Autodesk Inventor part; units mm, degrees
ref_plane "YZ Plane" through (0, 0, 0) normal (1, 0, 0) x (0, 1, 0)
ref_plane "XZ Plane" through (0, 0, 0) normal (0, 1, 0) x (-1, 0, 0)
ref_plane "XY Plane" through (0, 0, 0) normal (0, 0, 1) x (1, 0, 0)
sketch "Sketch1" plane through (0, 0, 0) normal (0, 1, 0) x (-1, 0, 0)
  line L0 (0, 0) -> (7, 0)
  line L1 (7, -23.495) -> (0, -23.495)
  line L2 (-11.75, -2) -> (-11.75, -21.5)
  line L3 (-11.75, -9.75) -> (-10, -9.75)
  line L4 (-10, -2) -> (-10, -21.5)
  line L5 (-11.75, -0.1283) -> (-10, -0.1283)
  line L6 (-10, -2) -> (-10, -6)
  line L7 (-11.75, -6) -> (-13.75, -6)
  line L8 (-13.75, -6) -> (-13.75, 0)
  line L9 (-10, -6) -> (-8, -6)
  line L10 (-8, -6) -> (-8, 0)
  line L11 (-8, 0) -> (-13.75, 0)
  line L12 (-10, -21.5) -> (-10, -17.5)
  line L13 (-10, -17.5) -> (-8, -17.5)
  line L14 (-8, -17.5) -> (-8, -23.5)
  line L15 (-10, -2) -> (-11.75, -2)
  line L16 (-11.75, -6) -> (-11.75, -2)
  line L17 (-10, -21.5) -> (-11.75, -21.5)
  line L18 (-11.75, -21.5) -> (-11.75, -17.5)
  line L19 (-11.75, -17.5) -> (-13.75, -17.5)
  line L20 (-13.75, -17.5) -> (-13.75, -23.5)
  line L21 (-13.75, -23.5) -> (-8, -23.5)
  line L22 (-0.01, -3.75) -> (7, -3.75)
  line L23 (-8, -6) -> (-0.01, -3.75)
  line L24 (-8, 0) -> (7, 0)
  line L25 (7, 0) -> (7, -3.75)
  line L26 (-8, -23.5) -> (7, -23.5)
  line L27 (7, -23.5) -> (7, -19.75)
  line L28 (7, -19.75) -> (-0.01, -19.75)
  line L29 (-8, -17.5) -> (-0.01, -19.75)
  line L30 (7, -23.5) -> (0, -23.5)
  line L31 (0, -23.5) -> (0, 0)
  line L32 (0, 0) -> (7, 0)
  line L33 (7, 0) -> (7, -23.5)
  line L34 (-10, -21.5) -> (-9.75, -21.5)
  line L35 (-9.75, -21.5) -> (-9.75, -17.5)
  line L36 (-9.75, -17.5) -> (-10, -17.5)
  line L37 (-10, -17.5) -> (-10, -21.5)
  line L38 (-11.75, -17.5) -> (-12, -17.5)
  line L39 (-12, -17.5) -> (-12, -21.5)
  line L40 (-12, -21.5) -> (-11.75, -21.5)
  line L41 (-11.75, -21.5) -> (-11.75, -17.5)
  line L42 (-10, -6) -> (-9.75, -6)
  line L43 (-9.75, -6) -> (-9.75, -2)
  line L44 (-9.75, -2) -> (-10, -2)
  line L45 (-10, -2) -> (-10, -6)
  line L46 (-11.75, -6) -> (-12, -6)
  line L47 (-12, -6) -> (-12, -2)
  line L48 (-12, -2) -> (-11.75, -2)
  line L49 (-11.75, -2) -> (-11.75, -6)
  dimension "d0" = 23.495
  dimension "d1" = 7
  dimension "d2" = 4
  dimension "d3" = 2
  dimension "d4" = 6
  dimension "d5" = 2
  dimension "d6" = 4
  dimension "d7" = 2
  dimension "d8" = 6
  dimension "d9" = 2
  dimension "d10" = 15
  dimension "d11" = 15
  dimension "d12" = 0.25
  dimension "d13" = 0.25
  dimension "d14" = 0.25
  dimension "d15" = 0.25
extrude "Extrusion1" add sketch "Sketch1" along normal blind 14.5 contours L31 L22 L23 L10 L24 | L0 L25 L22 L31 | L10 L9 L43 L44 L15 L48 L47 L7 L8 L11 | L22 L33 L28 L31 | L31 L26 L14 L29 L28 | L28 L27 L1 L31 | L1 L27 L26 L31 | L14 L21 L20 L19 L39 L40 L17 L34 L35 L13
sketch "Sketch2" plane through (-7, 0, -23.5) normal (-1, 0, 0) x (0, 0, 1)
  line L0 (23.5, 0) -> (19.75, 0)
  line L1 (19.75, 0) -> (3.75, 0)
  line L2 (19.75, 0) -> (19.75, 14.5)
  line L3 (19.75, 0) -> (19.75, 14.5)
  line L4 (6, 0) -> (0, 0)
  line L5 (0, 0) -> (3.75, 0)
  line L6 (3.75, 0) -> (3.75, 14.5)
  line L7 (3.75, 0) -> (3.75, 14.5)
  line L8 (3.75, 0) -> (19.75, 0)
  line L9 (19.75, 0) -> (19.75, 14.5)
  line L10 (19.75, 14.5) -> (3.75, 14.5)
  line L11 (3.75, 14.5) -> (3.75, 0)
  dimension "d18" = 3.75
  dimension "d19" = 3.75
extrude "Extrusion2" add sketch "Sketch2" along normal blind 30
sketch "Sketch3" plane through (0, 0, 0) normal (0, -1, 0) x (1, 0, 0)
  line L0 (-37, -19.75) -> (-37, -3.75)
  circle A0 centre (-37, -11.75) radius 10.75
  point P0 (0, 0)
  dimension "d22" = 21.5
extrude "Extrusion3" add sketch "Sketch3" against normal blind 14.5
sketch "Sketch4" plane through (0, 0, 0) normal (0, -1, 0) x (1, 0, 0)
  arc A0 (-29.8193, -3.75) -> (-29.8193, -19.75) centre (-37, -11.75) ccw
  circle A1 centre (-37, -11.75) radius 10
  point P0 (0, 0)
  dimension "d25" = 20
extrude "Extrusion4" cut sketch "Sketch4" against normal blind 10.5
sketch "Sketch5" plane through (-37, 10.5, -11.75) normal (0, -1, 0) x (1, 0, 0)
  circle A0 centre (0, 0) radius 10
  circle A1 centre (0, 0) radius 9.5
  point P0 (37, 11.75)
  dimension "d28" = 19
extrude "Extrusion5" cut sketch "Sketch5" against normal blind 10.5 contours A1
sketch "Sketch6" plane through (0, 0, -3.75) normal (1, 0, 0) x (0, 0, -1)
  circle A0 centre (8, 7.25) radius 5.25
  point P0 (-3.75, 0)
  dimension "d31" = 10.5
extrude "Extrusion6" cut sketch "Sketch6" against normal blind 40
sketch "Sketch7" plane through (0, 14.5, 0) normal (0, 1, 0) x (1, 0, 0)
  arc A0 (-29.8193, 19.75) -> (-29.8193, 3.75) centre (-37, 11.75) ccw
  circle A1 centre (-37, 11.75) radius 10.75
  point P0 (0, 0)
  dimension "d50" = 21.5
extrude "Extrusion7" cut sketch "Sketch7" against normal blind 1
sketch "Sketch9" plane through (0, 0, 0) normal (0, -1, 0) x (1, 0, 0)
  line L0 (-7, -19.75) -> (-29.8193, -19.75)
  line L1 (-7, -19.75) -> (-4, -19.75)
  line L2 (-4, -19.75) -> (-4, -16.75)
  line L3 (-7, -3.75) -> (-7, 0)
  line L4 (-7, -3.75) -> (-4, -3.75)
  line L5 (-4, -3.75) -> (-4, -6.75)
  line L6 (-4, -16.75) -> (-24, -16.75)
  line L7 (-24, -16.75) -> (-24, -6.75)
  line L8 (-24, -6.75) -> (-4, -6.75)
  line L9 (-4, -6.75) -> (-4, -16.75)
  point P0 (0, 0)
  point P1 (-29.0904, -19.75)
  dimension "d39" = 3
  dimension "d40" = 3
  dimension "d41" = 3
  dimension "d42" = 3
  dimension "d43" = 20
extrude "Extrusion9" cut sketch "Sketch9" against normal blind 3
sketch "Sketch10" plane through (0, 3, 0) normal (0, -1, 0) x (1, 0, 0)
  line L0 (-4, -8.6678) -> (-24, -8.6678)
  line L1 (-4, -6.75) -> (-4, -8.6678)
  line L2 (-24, -6.75) -> (-4, -6.75)
  line L3 (-24, -8.6678) -> (-24, -6.75)
  line L4 (-24, -14.8322) -> (-4, -14.8322)
  line L5 (-24, -16.75) -> (-24, -14.8322)
  line L6 (-4, -16.75) -> (-24, -16.75)
  line L7 (-4, -14.8322) -> (-4, -16.75)
  point P0 (0, 0)
extrude "Extrusion10" add sketch "Sketch10" along normal blind 3
sketch "Sketch11" plane through (13.75, 0, -17.5) normal (1, 0, 0) x (0, 0, -1)
  line L0 (-15.5, 11.975) -> (4, 11.975)
  line L1 (4, 0) -> (4, 14.5)
  line L2 (4, 11.975) -> (4, 14.5)
  line L3 (4, 14.5) -> (-15.625, 14.5)
  line L4 (-13.75, 14.5) -> (-17.5, 14.5)
  line L5 (-15.5, 0) -> (-15.5, 14.5)
  line L6 (-15.5, 11.975) -> (-15.5, 14.5)
  line L7 (4, 11.975) -> (-15.5, 11.975)
  line L8 (-15.5, 14.5) -> (4, 14.5)
  point P0 (-17.5, 0)
extrude "Extrusion11" add sketch "Sketch11" against normal blind 5.75
properties part number "PistonV2"
Check sheet for the modelled part. Datum: model origin and axes. Units: mm. A direction names the side the tool comes from. Give positions to 0.01 mm unless a question says otherwise; leave off trailing zeros. Order: outer loops, then holes, each group sorted by start corner. A loop starts at its lowest first (then second) coordinate and runs counter-clockwise, first axis right, second up. Notation, with made-up numbers: (25, 30.25) -> (56, 30.25) arc R18 cw to (56, 34.25) -> close; hole circle Ø1 at (32, 55.25). An arc over 180 degrees is marked (long way). Return JSON: item names as keys, results as strings.
1. Material ranges on probe 1 along Z at (x, y) = (-20, 3); probe 2 along Z at (x, y) = (-37, 12.15); probe 3 along X at (y, z) = (1.75, -3) (3 decimals), recorded low to high. Write a range as [from, to].
From the geometry:
{"probe 1": "[-19.75, -14.83], [-8.67, -3.75]", "probe 2": "[-22.5, -21.25], [-2.25, -1]", "probe 3": "[-43.245, -41.841], [-32.159, -30.755], [-7, 9.75], [12, 13.75]"}
2. Cross-section at A-A, the plane x = -37. Record the cut outline in (y, z).
From the geometry:
{"outline": "(0, -22.5) -> (13.5, -22.5) -> (13.5, -21.25) -> (10.5, -21.25) -> (10.5, -21.75) -> (0, -21.75) -> close; (0, -1.75) -> (10.5, -1.75) -> (10.5, -2.25) -> (13.5, -2.25) -> (13.5, -1) -> (0, -1) -> close"}
3. Mould release check, pull along X, two halves, no side actions. Record for faces 4 (the flat face through (13, 6, -17.5)), 5 (the cylindrical face through (-26.25, 14.01, -11.62)), 6 (the flat face through (-14, 2, -14.832)): +X half, -X half, draft (parallel to the pull), parting line (faces both ways), or undercut.
From the geometry:
{"face 4": "draft", "face 5": "-X half", "face 6": "undercut"}
4. Cross-section at B-B, the plane z = -11.75. Record the cut outline in (x, y) (3 decimals), plus the area to 3 significant figures.
From the geometry:
{"outline": "(-47.75, 0) -> (-47, 0) -> (-47, 10.5) -> (-46.5, 10.5) -> (-46.5, 13.5) -> (-47.75, 13.5) -> close; (-27.5, 12.5) -> (0, 12.5) -> (0, 14.5) -> (-26.25, 14.5) -> (-26.25, 13.5) -> (-27.5, 13.5) -> close; (-27, 0) -> (-24, 0) -> (-24, 2) -> (-27, 2) -> close; (-4, 0) -> (0, 0) -> (0, 2) -> (-4, 2) -> close; (8, 11.975) -> (13.75, 11.975) -> (13.75, 14.5) -> (8, 14.5) -> close", "area": "93.9 mm^2"}
5. Set-up check for faces 1 (the flat face through (-18, 7, -19.75)), 2 (the flat face through (-14, 2, -8.668)), 3 (the flat face through (4.1, 7.1, -4.9)): record each of +Z, -Z, +X, -X, +Y, -Y from which the full face is reachable in a straight line by a thin tool's end or side.
From the geometry:
{"face 1": "-Z, +Y, -Y", "face 2": "-Y", "face 3": "+Y, -Y"}
6. Go/stop test with flat-tipped pins: P1, Ø4.5, axis at y = 3.5, z = -10, coming from the +X side; P2, Ø3, axis at y = 11, z = -16, coming from the -X side; P3, Ø3, axis at y = 13, z = -9, coming from the -X side. Record where each tip stops, or that it passes through.
From the geometry:
{"P1": "x = 0", "P2": "x = -47.39", "P3": "x = -47.68"}
